Autodesk Inventor part; units mm, degrees
ref_plane "YZ Plane" through (0, 0, 0) normal (1, 0, 0) x (0, 1, 0)
ref_plane "XZ Plane" through (0, 0, 0) normal (0, 1, 0) x (-1, 0, 0)
ref_plane "XY Plane" through (0, 0, 0) normal (0, 0, 1) x (1, 0, 0)
sketch "Sketch1" plane through (0, 0, 0) normal (0, 0, 1) x (1, 0, 0)
  circle A0 centre (0, 0) radius 1.5
  circle A1 centre (0, 0) radius 4.5
  dimension "d0" = 3
  dimension "d1" = 9
extrude "Extrusion1" add sketch "Sketch1" along normal blind 8.6
sketch "Sketch2" plane through (0, 0, 8.6) normal (0, 0, 1) x (1, 0, 0)
  circle A0 centre (0, 0) radius 6.5
  circle A1 centre (0, 0) radius 1.5
  dimension "d4" = 13
extrude "Extrusion2" add sketch "Sketch2" against normal blind 1
sketch "Sketch3" plane through (0, 0, 0) normal (0, 0, -1) x (-1, 0, 0)
  circle A0 centre (0, 0) radius 6.5
  circle A1 centre (0, 0) radius 4.5
  circle A2 centre (0, 0) radius 4.5
  circle A3 centre (0, 0) radius 1.5
extrude "Extrusion3" add sketch "Sketch3" against normal blind 1 contours A0 | A1
ref_plane "Work Plane1" through (0, 0, 4.3) normal (0, 0, 1) x (1, 0, 0)
properties part number "belt pulley flanged"
The model under review builds one solid part; all positions refer to its coordinate system, in mm. A direction names the side the tool comes from. Give positions to 0.01 mm unless a question says otherwise; leave off trailing zeros. Order: outer loops, then holes, each group sorted by start corner. A loop starts at its lowest first (then second) coordinate and runs counter-clockwise, first axis right, second up. Notation, with made-up numbers: (-29, -11) -> (4, -11) arc R16 ccw to (4, 9) -> close; hole circle Ø6 at (40.25, 70.25). An arc over 180 degrees is marked (long way). Write item = value, one per line. Start each with the question number.
(1) Draft analysis for pull direction X (two halves, no side actions). For faces 1 (the cylindrical face through (-5.158, -3.955, 8.107)), 2 (the flat face through (1.54, 4.42, 1)), 3 (the cylindrical face through (-1.5, -0.07, 4.24)), state which applies: +X half, -X half, draft (parallel to the pull), parting line (faces both ways), or undercut.
(2) Take a section at C-C (z = 2.25). Write out the cut boundary in (x, y), plus the area to 3 significant figures.
(3) For L1, parallel to Z at x = 4.5, y = -1.75; L2, parallel to Y at x = 0, z = 3.5; L3, parallel to X at y = 2.25, z = 5, list the stretches that pass through material, from the lowest coordinate up. Write a range as from..to.
(4) Take a section at A-A (y = 0). Write out the cut boundary in (x, z).
(5) Tool access review of faces 4 (the cylindrical face through (5.158, -3.955, 0.493)), 5 (the flat face through (-1.54, 4.42, 7.6)): name each direction out of +Z, -Z, +X, -X, +Y, -Y from which nothing blocks a thin tool from reaching the whole face with its end or side.
(6) Take a section at D-D (x = -3). Write out the cut boundary in (y, z), plus the area to 3 significant figures.
(7) For pin 1 Ø3 at (x, z) = (1, 5) entering from +Y; pin 2 Ø1 at (x, z) = (2.5, 7.5) entering from +Y, all flat-tipped, find the tip position at first contact; note any pin that passes through.
Returned:
q1.face_1 = parting line
q1.face_2 = draft
q1.face_3 = undercut
q2.outline = circle Ø9 at (0, 0); hole circle Ø3 at (0, 0)
q2.area = 56.5 mm²
q3.L1 = 0..1, 7.6..8.6
q3.L2 = -4.5..-1.5, 1.5..4.5
q3.L3 = -3.9..3.9
q4.outline = (-6.5, 0) -> (-1.5, 0) -> (-1.5, 8.6) -> (-6.5, 8.6) -> (-6.5, 7.6) -> (-4.5, 7.6) -> (-4.5, 1) -> (-6.5, 1) -> close; (1.5, 0) -> (6.5, 0) -> (6.5, 1) -> (4.5, 1) -> (4.5, 7.6) -> (6.5, 7.6) -> (6.5, 8.6) -> (1.5, 8.6) -> close
q5.face_4 = +Z, -Z
q5.face_5 = none
q6.outline = (-5.77, 0) -> (5.77, 0) -> (5.77, 1) -> (3.35, 1) -> (3.35, 7.6) -> (5.77, 7.6) -> (5.77, 8.6) -> (-5.77, 8.6) -> (-5.77, 7.6) -> (-3.35, 7.6) -> (-3.35, 1) -> (-5.77, 1) -> close
q6.area = 67.3 mm²
q7.pin_1 = 4.5
q7.pin_2 = 6.18
